```python
from build123d import *

# Parameters (mm, degrees)
F0_W     = 26.3
F0_H     = 26.3
F1_DEPTH = 11
F2_R     = 4
F3_R     = 7
F4_DEPTH = 18
F5_R     = 1.75
F5_R_2   = 0.75
F6_DEPTH = 2
F7_R     = 1.75
F7_R_2   = 0.75
F8_DEPTH = 2
F9_R     = 1


with BuildPart() as f1:
    # F0 (on Top) → F1 (new body)
    with BuildSketch(Plane.XY):
        with Locations((13.15, -13.15)):
            Rectangle(F0_W, F0_H)
    extrude(amount=F1_DEPTH)

    # F2
    f2_edges = [f1.edges().sort_by_distance(p)[0] for p in [
        (13.15, -26.3, 11),
        (0, -13.15, 11),
        (26.3, -13.15, 11),
        (13.15, 0, 11),
    ]]
    fillet(f2_edges, radius=F2_R)

    # F3 (on face) → F4 (join)
    with BuildSketch(Plane.XY.offset(11)):
        with Locations((13.15, -13.15)):
            Circle(F3_R)
    extrude(amount=F4_DEPTH)

    # F5 (on face) → F6 (join)
    with BuildSketch(Plane.XZ.offset(26.3)):
        with Locations((13.15, 4)):
            Circle(F5_R)
        with Locations((13.15, 4)):
            Circle(F5_R_2, mode=Mode.SUBTRACT)
    extrude(amount=F6_DEPTH)

    # F7 (on face) → F8 (join)
    with BuildSketch(Plane(origin=(0, 0, 0), x_dir=(-1, 0, 0), z_dir=(0, 1, 0))):
        with Locations((-13.15, 4)):
            Circle(F7_R)
        with Locations((-13.15, 4)):
            Circle(F7_R_2, mode=Mode.SUBTRACT)
    extrude(amount=F8_DEPTH)

    # F9
    f9_edges = [f1.edges().sort_by_distance(p)[0] for p in [
        (6.15, -13.15, 29),
    ]]
    fillet(f9_edges, radius=F9_R)


solid = f1.part
```
Model file for the job. Use its own axes, mm. A direction names the side the tool comes from. Round coordinates to 2 decimals unless told otherwise and drop trailing zeros. Loops run counter-clockwise (first coordinate to the right, second up) from the corner with the lowest first, then second, coordinate; pieces in that order, holes last. Notation, with made-up numbers: M 73,22 L 129,22 A28 cw 129,41 Z; hole C 17,-36.75 d5. An arc over 180 degrees is marked long. Put each result on its own line as item: value. Start each with the question number.
Item 1: Drill centre lines: line 1 along Z through (x, y) = (13.15, 1.1); line 2 along Z through (x, y) = (12.25, -22.5) (3 decimals); line 3 along Y through (x, z) = (15.25, 7.25). Where is each one in solid material? Low to high.
Item 2: Cut at A-A (y = -13.15). List the corners of the cut face in (x, z).
Item 3: Drop flat-ended pins along their axis: P1, Ø4, axis at x = 12, z = 16.5, coming from the +Y side; P2, Ø0.9, axis at x = 13.15, z = 4, coming from the -Y side; P3, Ø2, axis at x = 22, y = -10, coming from the +Z side. Give the stop position or say it passes through.
Item 4: 3-axis set-ups, long thin cutter, end or side, ignore diameter. For faces 1 (the face through (13, 0, 4)), 2 (the face through (7, -17, 11)), 3 (the face through (12.77, -27.29, 2.29)): which of +Z, -Z, +X, -X, +Y, -Y reach the whole face in a straight line?
Item 5: Cut at B-B (z = 4). List the corners of the cut face in (x, y), then the cut area to 3 significant figures.
Item 6: Cut at C-C (x = 13.15). List the corners of the cut face in (y, z), then the cut area to 3 significant figures.
Item 7: Cut at D-D (x = 4.5). List the corners of the cut face in (y, z), then the cut area to 3 significant figures.
Item 8: Mould opens along X. For faces 4 (the face through (13.334, -25.159, 9.797)), 5 (the face through (13.84, -27.29, 3.71)), 6 (the face through (11.533, 0.986, 3.33)) say: released by +X, released by -X, zero draft, split by the parting line, or undercut.
Answer block:
1. line 1: 2.25 to 3.25, 4.75 to 5.75
1. line 2: 0 to 10.995
1. line 3: -26.29 to -0.01
2. outline: M 0,0 L 26.3,0 L 26.3,7 A4 ccw 22.3,11 L 20.15,11 L 20.15,28 A1 ccw 19.15,29 L 7.15,29 A1 ccw 6.15,28 L 6.15,11 L 4,11 A4 ccw 0,7 Z
3. P1: y = -6.15
3. P2: y = -26.3
3. P3: z = 11
4. face 1: +Y
4. face 2: +Z
4. face 3: -Y
5. outline: M 0,-26.3 L 11.4,-26.3 L 11.4,-28.3 L 12.4,-28.3 L 12.4,-26.3 L 13.9,-26.3 L 13.9,-28.3 L 14.9,-28.3 L 14.9,-26.3 L 26.3,-26.3 L 26.3,0 L 14.9,0 L 14.9,2 L 13.9,2 L 13.9,0 L 12.4,0 L 12.4,2 L 11.4,2 L 11.4,0 L 0,0 Z
5. area: 700 mm2
6. outline: M -28.3,2.25 L -26.3,2.25 L -26.3,0 L 0,0 L 0,2.25 L 2,2.25 L 2,3.25 L 0,3.25 L 0,4.75 L 2,4.75 L 2,5.75 L 0,5.75 L 0,7 A4 ccw -4,11 L -6.15,11 L -6.15,28 A1 ccw -7.15,29 L -19.15,29 A1 ccw -20.15,28 L -20.15,11 L -22.3,11 A4 ccw -26.3,7 L -26.3,5.75 L -28.3,5.75 L -28.3,4.75 L -26.3,4.75 L -26.3,3.25 L -28.3,3.25 Z
6. area: 542 mm2
7. outline: M -26.3,0 L 0,0 L 0,7 A4 ccw -4,11 L -22.3,11 A4 ccw -26.3,7 Z
7. area: 282 mm2
8. face 4: zero draft
8. face 5: undercut
8. face 6: split by the parting line
